Source: three-view drawing plus pictorial views. Frame: mm from the lowest corner of the part. Coordinates: 2 decimals unless noted, no trailing zeros. Write each loop counter-clockwise with the first axis right and the second up, starting at its lowest first coordinate (ties: lowest second). Pieces come first, ordered by that corner, then holes. Notation, with made-up numbers: (27.25, -7) - (47.25, -7) arc R33 cw to (47.25, 23) - close; hole circle Ø8 at (25, 55.25). An arc over 180 degrees is marked (long way). Answer as a JSON object with one key per item and string values. Group by question number.
Item 1: Section C-C on y = 22.75. Return loops of the section in (x, z), and give its area (3 significant figures).
Item 2: Section D-D on z = 2. Return loops of the section in (x, y).
Item 3: Section A-A on z = 15. Return loops of the section in (x, y).
Item 4: Mould query, pull axis X, two halves, no side actions, for the marked faces 1, 2 and 3. Classes: pulls with the +X half, pulls with the -X half, needs draft (parallel to the pull), parting line crosses it, or undercut.
Item 5: First-contact query: pin 1 Ø2 at (x, y) = (5, 5) entering from -Z. Flat tip, straight axial feed; report the tip coordinate or a pass-through.
Item 6: Line query: line 1 along Y through (x, z) = (5, 1.8); line 2 along Z through (x, y) = (17.5, 14.5); line 3 along X through (y, z) = (15.25, 16.5). Output: solid intervals per line, ascending. Write a range as from..to.
Item 7: Section B-B on x = 17. Return loops of the section in (y, z), and give its area (3 significant figures).
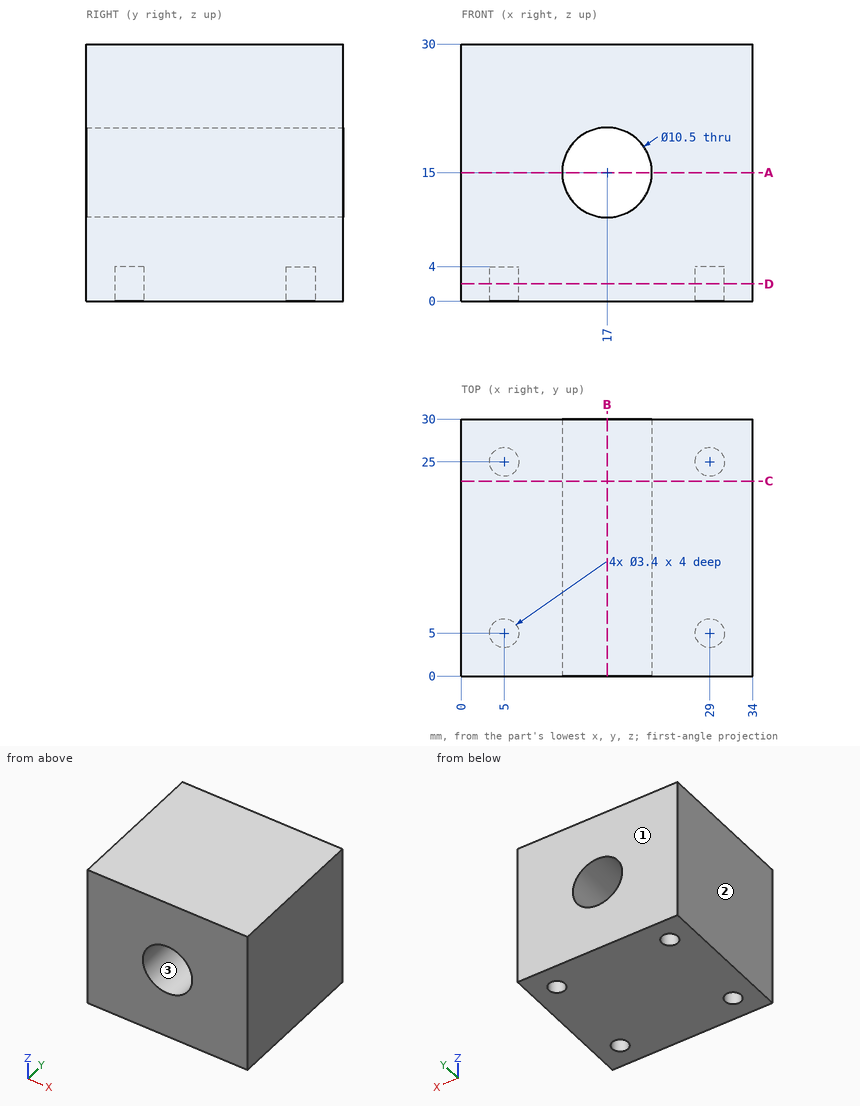
Checks:
{
 "1": {"outline": "(0, 0) - (34, 0) - (34, 30) - (0, 30) - close; hole circle Ø10.5 at (17, 15)", "area": "933 mm^2"},
 "2": {"outline": "(0, 0) - (34, 0) - (34, 30) - (0, 30) - close; hole circle Ø3.4 at (5, 5); hole circle Ø3.4 at (5, 25); hole circle Ø3.4 at (29, 5); hole circle Ø3.4 at (29, 25)"},
 "3": {"outline": "(0, 0) - (11.75, 0) - (11.75, 30) - (0, 30) - close; (22.25, 0) - (34, 0) - (34, 30) - (22.25, 30) - close"},
 "4": {"face 1": "needs draft", "face 2": "pulls with the -X half", "face 3": "undercut"},
 "5": {"pin 1": "z = 4"},
 "6": {"line 1": "0..3.3, 6.7..23.3, 26.7..30", "line 2": "0..9.77, 20.23..30", "line 3": "0..11.97, 22.03..34"},
 "7": {"outline": "(0, 0) - (30, 0) - (30, 9.75) - (0, 9.75) - close; (0, 20.25) - (30, 20.25) - (30, 30) - (0, 30) - close", "area": "585 mm^2"}
}
